```python
from build123d import *

# Parameters (mm, degrees)
SKETCH1_R             = 1.6
BOSS_EXTRUDE1_DEPTH   = 7
BOSS_EXTRUDE1_2_DEPTH = 7
BOSS_EXTRUDE1_3_DEPTH = 7
BOSS_EXTRUDE1_4_DEPTH = 7
BOSS_EXTRUDE2_DEPTH   = 2.5
SKETCH3_R             = 2.25
SKETCH3_R_2           = 0.75
BOSS_EXTRUDE3_DEPTH   = 3
SKETCH4_W             = 24.5
SKETCH4_H             = 6
BOSS_EXTRUDE4_DEPTH   = 2.5
CUT_EXTRUDE1_START    = -10
SKETCH5_R             = 0.75
CUT_EXTRUDE1_DEPTH    = 10


with BuildPart() as part:
    # Sketch1 → Boss-Extrude1 (new body)
    with BuildSketch(Plane(origin=(0, 0, 0), x_dir=(1, 0, 0), z_dir=(0, 1, 0))):
        with Locations(Location((-15.25, -15.25, 0), (0, 0, 270))):
            Circle(SKETCH1_R)
    extrude(amount=BOSS_EXTRUDE1_DEPTH)



with BuildPart() as body_2:
    # Sketch1 → Boss-Extrude1 2 (new body)
    with BuildSketch(Plane(origin=(0, 0, 0), x_dir=(1, 0, 0), z_dir=(0, 1, 0))):
        with Locations(Location((-15.25, 15.25, 0), (0, 0, 270))):
            Circle(SKETCH1_R)
    extrude(amount=BOSS_EXTRUDE1_2_DEPTH)


with BuildPart() as body_3:
    # Sketch1 → Boss-Extrude1 3 (new body)
    with BuildSketch(Plane(origin=(0, 0, 0), x_dir=(1, 0, 0), z_dir=(0, 1, 0))):
        with Locations(Location((15.25, 15.25, 0), (0, 0, 270))):
            Circle(SKETCH1_R)
    extrude(amount=BOSS_EXTRUDE1_3_DEPTH)


with BuildPart() as body_4:
    # Sketch1 → Boss-Extrude1 4 (new body)
    with BuildSketch(Plane(origin=(0, 0, 0), x_dir=(1, 0, 0), z_dir=(0, 1, 0))):
        with Locations(Location((15.25, -15.25, 0), (0, 0, 270))):
            Circle(SKETCH1_R)
    extrude(amount=BOSS_EXTRUDE1_4_DEPTH)


with BuildPart() as part_1:
    add(part.part)

    add(body_2.part)  # Boss-Extrude2 merges body 2

    add(body_3.part)  # Boss-Extrude2 merges body 3

    add(body_4.part)  # Boss-Extrude2 merges body 4
    # Sketch2 → Boss-Extrude2 (add)
    with BuildSketch(Plane.XZ):
        Polygon((-12.25, 12.25), (12.25, 12.25), (12.25, -18.25), (18.25, -18.25), (18.25, 19.25), (-18.25, 19.25), (-18.25, -18.25), (-12.25, -18.25), align=None)
    extrude(amount=BOSS_EXTRUDE2_DEPTH)

    # Sketch3 → Boss-Extrude3 (add)
    # profile 1 of 4: a face of its own
    with BuildSketch(Plane.XZ.offset(2.5)):
        with Locations(Location((-10.25, 16.25, 0), (0, 0, 90))):
            Circle(SKETCH3_R)
        with Locations(Location((-10.25, 16.25, 0), (0, 0, 270))):
            Circle(SKETCH3_R_2, mode=Mode.SUBTRACT)
    # profile 2 of 4: a face of its own
    with BuildSketch(Plane.XZ.offset(2.5)):
        with Locations(Location((10.25, 16.25, 0), (0, 0, 90))):
            Circle(SKETCH3_R)
        with Locations(Location((10.25, 16.25, 0), (0, 0, 270))):
            Circle(SKETCH3_R_2, mode=Mode.SUBTRACT)
    # profile 3 of 4: a face of its own
    with BuildSketch(Plane.XZ.offset(2.5)):
        with Locations(Location((10.25, -4.25, 0), (0, 0, 27.266044451))):
            Circle(SKETCH3_R)
        with Locations(Location((10.25, -4.25, 0), (0, 0, 270))):
            Circle(SKETCH3_R_2, mode=Mode.SUBTRACT)
    # profile 4 of 4: a face of its own
    with BuildSketch(Plane.XZ.offset(2.5)):
        with Locations(Location((-10.25, -4.25, 0), (0, 0, 152.733955549))):
            Circle(SKETCH3_R)
        with Locations(Location((-10.25, -4.25, 0), (0, 0, 270))):
            Circle(SKETCH3_R_2, mode=Mode.SUBTRACT)
    extrude(amount=BOSS_EXTRUDE3_DEPTH)

    # Sketch4 → Boss-Extrude4 (add)
    with BuildSketch(Plane(origin=(0, -2.5, 0), x_dir=(1, 0, 0), z_dir=(0, 1, 0))):
        with Locations((0, 4.25)):
            Rectangle(SKETCH4_W, SKETCH4_H)
    extrude(amount=BOSS_EXTRUDE4_DEPTH)

    # Sketch5 → Cut-Extrude1 (cut)
    with BuildSketch(Plane.XZ.offset(2.5).offset(CUT_EXTRUDE1_START)):
        with Locations(Location((-10.25, 16.25, 0), (0, 0, 90))):
            Circle(SKETCH5_R)
        with Locations(Location((10.25, 16.25, 0), (0, 0, 90))):
            Circle(SKETCH5_R)
        with Locations(Location((10.25, -4.25, 0), (0, 0, 90))):
            Circle(SKETCH5_R)
        with Locations(Location((-10.25, -4.25, 0), (0, 0, 90))):
            Circle(SKETCH5_R)
    extrude(amount=CUT_EXTRUDE1_DEPTH, mode=Mode.SUBTRACT)


solid = part_1.part
```
For this review, take the finished solid that the model builds, in its own axes (mm). A direction names the side the tool comes from. Round coordinates to 2 decimals unless told otherwise and drop trailing zeros. Write each loop counter-clockwise with the first axis right and the second up, starting at its lowest first coordinate (ties: lowest second). Pieces come first, ordered by that corner, then holes. Notation, with made-up numbers: (-27, 77) - (-2, 77) arc R17 ccw to (-2, 97) - close; hole circle Ø2 at (68.25, 10). An arc over 180 degrees is marked (long way). Put each result on its own line as item: value.
Q1. Insertion check: pin 1 Ø0.9 at (x, z) = (10.25, -4.25) entering from +Y; pin 2 Ø10 at (x, z) = (-10, -1) entering from +Y; pin 3 Ø11 at (x, z) = (-5.5, 1) entering from -Y; pin 4 Ø1.2 at (x, y) = (-2.5, -1) entering from -Z. Each pin has a flat end and moves straight along its axis. Give the tip position at first contact, or say it passes through.
Solved:
pin 1: passes through
pin 2: stops at y = 0
pin 3: stops at y = -5.5
pin 4: stops at z = -7.25
Q2. We need section C-C (z = -10). Give the boundary of the cut face in (x, y), and give its area (3 significant figures).
Solved:
outline: (-18.25, -2.5) - (-12.25, -2.5) - (-12.25, 0) - (-18.25, 0) - close; (12.25, -2.5) - (18.25, -2.5) - (18.25, 0) - (12.25, 0) - close
area: 30.0 mm2
Q3. We need section D-D (y = 3.25). Give the boundary of the cut face in (x, z), and give its area (3 significant figures).
Solved:
outline: circle Ø3.2 at (-15.25, -15.25); circle Ø3.2 at (-15.25, 15.25); circle Ø3.2 at (15.25, -15.25); circle Ø3.2 at (15.25, 15.25)
area: 32.2 mm2
Q4. We need section A-A (z = -4.25). Give the boundary of the cut face in (x, y).
Solved:
outline: (-18.25, -2.5) - (-12.5, -2.5) - (-12.5, -5.5) - (-11, -5.5) - (-11, 0) - (-18.25, 0) - close; (-9.5, -5.5) - (-8, -5.5) - (-8, -2.5) - (8, -2.5) - (8, -5.5) - (9.5, -5.5) - (9.5, 0) - (-9.5, 0) - close; (11, -5.5) - (12.5, -5.5) - (12.5, -2.5) - (18.25, -2.5) - (18.25, 0) - (11, 0) - close
Q5. Wall thickness on probe 1 along Z at (x, y) = (-10.25, -3.6); probe 2 along X at (y, z) = (-4.2, -4.25); probe 3 along X at (y, z) = (-1.15, 16.25): over which ranges is each line inside the solid? List them lowest first.
Solved:
probe 1: z = -6.5 to -5, -3.5 to -2, 14 to 15.5, 17 to 18.5
probe 2: x = -12.5 to -11, -9.5 to -8, 8 to 9.5, 11 to 12.5
probe 3: x = -18.25 to -11, -9.5 to 9.5, 11 to 18.25
Q6. Machinability: for faces 1 (the face through (0, -1, -1.25)), 2 (the face through (0, -1, -7.25)), 3 (the face through (16.33, 3.45, -16.43)), 4 (the face through (-10.926, -3.979, 18.396)), 5 (the face through (-15, -1, -18.25)), which of the approach directions +Z, -Z, +X, -X, +Y, -Y give a long, thin tool a straight path to every point of the face, cutting with its end or side? Answer none if there is none.
Solved:
face 1: +Y, -Y
face 2: -Z, +Y, -Y
face 3: +Y
face 4: -Y
face 5: -Z, +X, -X, +Y, -Y
Q7. We need section B-B (x = -10.25). Give the boundary of the cut face in (y, z), and give its area (3 significant figures).
Solved:
outline: (-5.5, -6.5) - (-2.5, -6.5) - (-2.5, -7.25) - (0, -7.25) - (0, -5) - (-5.5, -5) - close; (-5.5, -3.5) - (0, -3.5) - (0, -1.25) - (-2.5, -1.25) - (-2.5, -2) - (-5.5, -2) - close; (-5.5, 14) - (-2.5, 14) - (-2.5, 12.25) - (0, 12.25) - (0, 15.5) - (-5.5, 15.5) - close; (-5.5, 17) - (0, 17) - (0, 19.25) - (-2.5, 19.25) - (-2.5, 18.5) - (-5.5, 18.5) - close
area: 43.0 mm2
Q8. Mouldability with a two-part tool opening along X and no side actions: class faces 6 (the face through (12.25, -1, 6)), 7 (the face through (-15, 7, -15)), 8 (the face through (-18.25, -1, 1)) as released by +X, released by -X, zero draft, split by the parting line, or undercut.
Solved:
face 6: undercut
face 7: zero draft
face 8: released by -X
